Read the model definition and answer for the solid it produces. Units are mm, in the model's axes. Face numbers are marked on the shaded views. A direction names the side the tool comes from. Round coordinates to 2 decimals unless told otherwise and drop trailing zeros. Order: outer loops, then holes, each group sorted by start corner. A loop starts at its lowest first (then second) coordinate and runs counter-clockwise, first axis right, second up. Notation, with made-up numbers: (26, -16.5) -> (43, -16.5) arc R13 ccw to (43, -1.5) -> close; hole circle Ø1 at (-13.5, -13.75). An arc over 180 degrees is marked (long way). Use a Markdown table: item, result. Add a question column.
1. Section B-B, the plane z = -12 is taken. Give the vertices of the cut face in (x, y).
2. Given pin 1 (0.5 mm diameter, centred on x = 10.5, z = 57.5, fed in from +Y); pin 2 (1 mm diameter, centred on x = 4.5, z = 32, fed in from +Y); pin 3 (2.5 mm diameter, centred on x = -1, y = 10, fed in from +Z); pin 4 (1 mm diameter, centred on x = 1.5, z = 50, fed in from -Y), each flat-ended and moving along its own axis, determine where each tip first touches the part or whether it passes through.
3. Consider L1, parallel to Y at x = 0, z = 1.9; L2, parallel to X at y = 7.75, z = 1.3; L3, parallel to X at y = -7, z = 2. Determine where each line is inside the solid, lowest interval first. Write a range as [from, to].
4. Section A-A, the plane z = 17 is taken. Give the vertices of the cut face in (x, y), then the cut area to 3 significant figures.
5. For the marked faces 1, 2, 3, 4 and 5, determine the directions among +Z, -Z, +X, -X, +Y, -Y from which every point of the face is accessible in a straight line to the end or side of a thin tool.
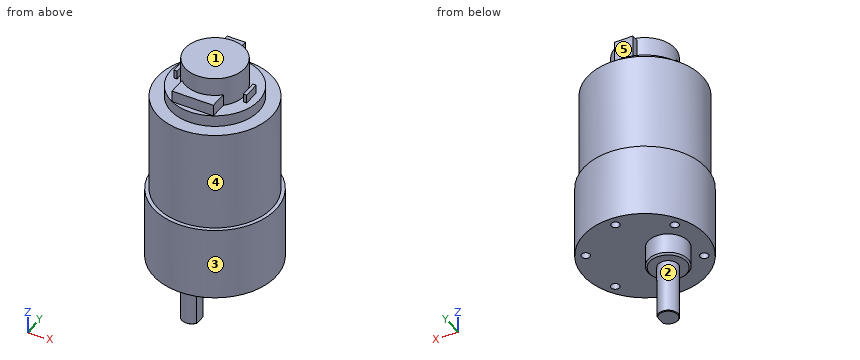
```python
from build123d import *

# Parameters (mm, degrees)
SKETCH1_R                   = 17.272
BOSS_EXTRUDE1_DEPTH         = 52.22
SKETCH1_3_R                 = 6
BOSS_EXTRUDE2_DEPTH         = 6.5
BOSS_EXTRUDE3_DEPTH         = 22.86
SKETCH1_5_R                 = 3
BOSS_EXTRUDE4_DEPTH         = 10.668
SKETCH2_W                   = 1
SKETCH2_H                   = 5
BOSS_EXTRUDE5_DEPTH         = 6
SKETCH4_R                   = 18.4
BOSS_EXTRUDE6_DEPTH         = 22
TAP_DRILL_FOR_M3_TAP1_D     = 2.5
TAP_DRILL_FOR_M3_TAP1_DEPTH = 3
TAP_DRILL_FOR_M3_TAP1_TIP   = 0.751075774
SKETCH9_R                   = 13.2715
BOSS_EXTRUDE7_DEPTH         = 3.429
SKETCH10_R                  = 8.97255
BOSS_EXTRUDE8_DEPTH         = 8.9154
SKETCH11_W                  = 12.446
SKETCH11_H                  = 6.0452
BOSS_EXTRUDE9_DEPTH         = 3.4544
SKETCH12_W                  = 5.4864
SKETCH12_H                  = 2.2098
BOSS_EXTRUDE10_DEPTH        = 7.874
CHAMFER1_SIZE               = 0.2
CHAMFER2_SIZE               = 0.5


with BuildPart() as part:
    # Sketch1 → Boss-Extrude1 (new body)
    with BuildSketch(Plane.XY):
        Circle(SKETCH1_R)
    extrude(amount=BOSS_EXTRUDE1_DEPTH)

    # Sketch1_3 → Boss-Extrude2 (add)
    with BuildSketch(Plane.XY):
        with Locations((-7, 0)):
            Circle(SKETCH1_3_R)
    extrude(amount=-BOSS_EXTRUDE2_DEPTH)

    # Sketch1_4 → Boss-Extrude3 (add)
    with BuildSketch(Plane.XY):
        with BuildLine():
            Line((-4.6, -1.8), (-4.6, 1.8))
            ThreePointArc((-4.6, 1.8), (-10, 0), (-4.6, -1.8))
        make_face()
    extrude(amount=-BOSS_EXTRUDE3_DEPTH)

    # Sketch1_5 → Boss-Extrude4 (add)
    with BuildSketch(Plane.XY):
        with Locations((-7, 0)):
            Circle(SKETCH1_5_R)
    extrude(amount=-BOSS_EXTRUDE4_DEPTH)

    # Sketch2 → Boss-Extrude5 (add)
    with BuildSketch(Plane.XY.offset(52.22)):
        with Locations((-10.5, 0)):
            Rectangle(SKETCH2_W, SKETCH2_H)
        with Locations((10.5, 0)):
            Rectangle(SKETCH2_W, SKETCH2_H)
    extrude(amount=BOSS_EXTRUDE5_DEPTH)

    # Sketch4 → Boss-Extrude6 (add)
    with BuildSketch(Plane(origin=(0, 0, 0), x_dir=(-1, 0, 0), z_dir=(0, 0, -1))):
        Circle(SKETCH4_R)
    extrude(amount=-BOSS_EXTRUDE6_DEPTH)

    # Tap Drill for M3 Tap1
    with Locations(Plane(origin=(0, 0, 0), x_dir=(-1, 0, 0), z_dir=(0, 0, -1))):
        with Locations((-13.423393759, -7.75), (0, -15.5), (0, 15.5), (13.423393759, 7.75), (13.423393759, -7.75), (-13.423393759, 7.75)):
            Hole(TAP_DRILL_FOR_M3_TAP1_D / 2, depth=TAP_DRILL_FOR_M3_TAP1_DEPTH)
            with Locations((0, 0, -(TAP_DRILL_FOR_M3_TAP1_DEPTH + TAP_DRILL_FOR_M3_TAP1_TIP / 2))):  # 118° drill point
                Cone(0, TAP_DRILL_FOR_M3_TAP1_D / 2, TAP_DRILL_FOR_M3_TAP1_TIP, mode=Mode.SUBTRACT)

    # Sketch9 → Boss-Extrude7 (add)
    with BuildSketch(Plane.XY.offset(52.22)):
        Circle(SKETCH9_R)
    extrude(amount=BOSS_EXTRUDE7_DEPTH)

    # Sketch10 → Boss-Extrude8 (add)
    with BuildSketch(Plane.XY.offset(55.649)):
        Circle(SKETCH10_R)
    extrude(amount=BOSS_EXTRUDE8_DEPTH)

    # Sketch11 → Boss-Extrude9 (add)
    with BuildSketch(Plane.XY.offset(55.649)):
        with Locations((0, -8.699472481)):
            Rectangle(SKETCH11_W, SKETCH11_H)
    extrude(amount=BOSS_EXTRUDE9_DEPTH)

    # Sketch12 → Boss-Extrude10 (add)
    with BuildSketch(Plane.XY.offset(55.649)):
        with Locations((0, 10.0584)):
            Rectangle(SKETCH12_W, SKETCH12_H)
    extrude(amount=BOSS_EXTRUDE10_DEPTH)

    # Chamfer1
    chamfer1_edges = [part.edges().sort_by_distance(p)[0] for p in [
        (-10, 0, -22.86),
    ]]
    chamfer(chamfer1_edges, length=CHAMFER1_SIZE)

    # Chamfer2
    chamfer2_edges = [part.edges().sort_by_distance(p)[0] for p in [
        (-13, 0, -6.5),
    ]]
    chamfer(chamfer2_edges, length=CHAMFER2_SIZE)


solid = part.part
```
Verdict:
| question | item | result |
|---|---|---|
| 1 | outline | (-4.6, -1.8) -> (-4.6, 1.8) arc R3 ccw (long way) to start |
| 2 | pin 1 | stops at y = 2.5 |
| 2 | pin 2 | stops at y = 16.8 |
| 2 | pin 3 | stops at z = 64.56 |
| 2 | pin 4 | stops at y = -17.24 |
| 3 | L1 | y = [-18.4, -16.75], [-14.25, 14.25], [16.75, 18.4] |
| 3 | L2 | x = [-16.69, -14.67], [-12.17, 12.17], [14.67, 16.69] |
| 3 | L3 | x = [-17.02, -14.42], [-12.42, 12.42], [14.42, 17.02] |
| 4 | outline | circle Ø36.8 at (0, 0) |
| 4 | area | 1,060 mm2 |
| 5 | face 1 | +Z, +X, -X, +Y, -Y |
| 5 | face 2 | -Z |
| 5 | face 3 | +Z, -Z |
| 5 | face 4 | +Z |
| 5 | face 5 | +Z, +X, -X, +Y |
